Source: three-view drawing plus pictorial views. Frame: mm from the lowest corner of the part. Coordinates: 2 decimals unless noted, no trailing zeros. Write each loop counter-clockwise with the first axis right and the second up, starting at its lowest first coordinate (ties: lowest second). Pieces come first, ordered by that corner, then holes. Notation, with made-up numbers: M 13,22.25 L 19,22.25 A33 ccw 19,57.25 Z; hole C -29,21 d9. An arc over 180 degrees is marked long. Write item = value, one per line. Start each with the question number.
Item 1: Section B-B on z = 1.3. Output: boundary loops of the cut face in (x, y), plus the area to 3 significant figures.
Item 2: Section A-A on x = 14.5. Output: boundary loops of the cut face in (y, z), plus the area to 3 significant figures.
Item 3: First-contact query: pin 1 Ø1.5 at (x, z) = (55, 2) entering from -Y. Flat tip, straight axial feed; report the tip coordinate or a pass-through.
Item 4: Section C-C on x = 80. Output: boundary loops of the cut face in (y, z).
Item 5: Ray query, L1, parallel to Y at x = 104.5, z = 0.55; L2, parallel to X at y = 80, z = 0.1; L3, parallel to Y at x = 85, z = 0.8. Return the intervals inside material, ascending. Write a range as [from, to].
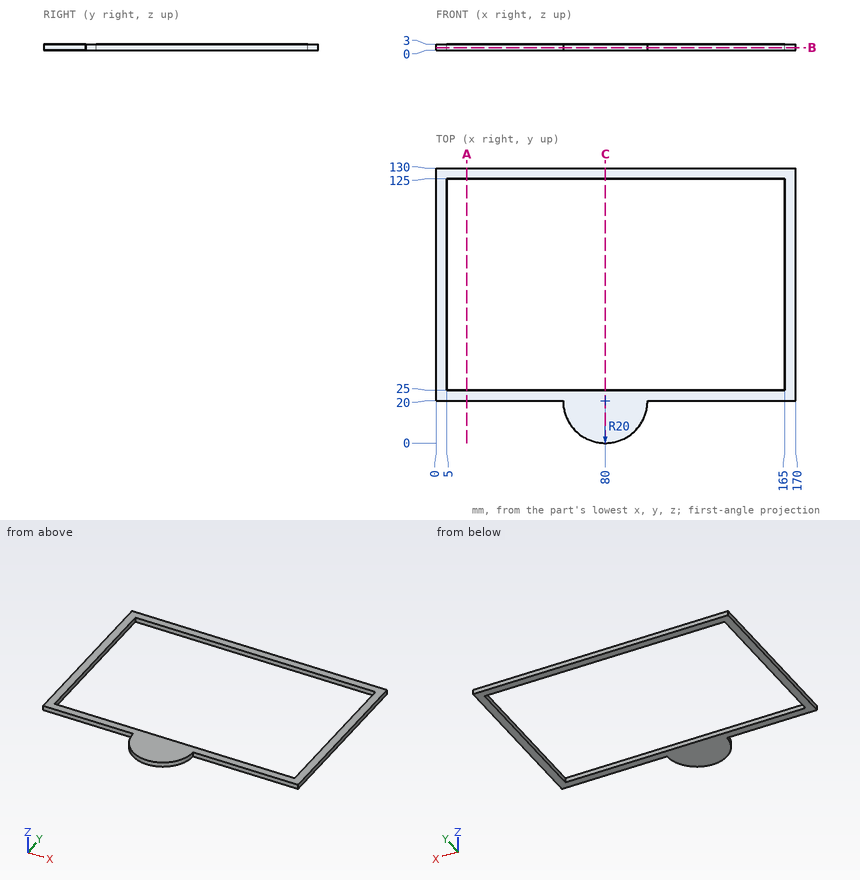
Responses:
q1.outline = M 0,20 L 60,20 A20 ccw 100,20 L 170,20 L 170,130 L 0,130 Z; hole M 5,25 L 165,25 L 165,125 L 5,125 Z
q1.area = 3,330 mm²
q2.outline = M 20,0 L 25,0 L 25,3 L 20,3 Z; M 125,0 L 130,0 L 130,3 L 125,3 Z
q2.area = 30.0 mm²
q3.pin_1 = 20
q4.outline = M 0,0 L 25,0 L 25,3 L 0,3 Z; M 125,0 L 130,0 L 130,3 L 125,3 Z
q5.L1 = [20, 25], [125, 130]
q5.L2 = [0, 5], [165, 170]
q5.L3 = [0.64, 25], [125, 130]
